Check sheet for the modelled part. Datum: model origin and axes. Units: mm. Face numbers are marked on the shaded views. A direction names the side the tool comes from. Coordinates: 2 decimals unless noted, no trailing zeros. Loops run counter-clockwise (first coordinate to the right, second up) from the corner with the lowest first, then second, coordinate; pieces in that order, holes last. Notation, with made-up numbers: (22.5, -16) -> (61.5, -16) arc R24 cw to (61.5, 6) -> close; hole circle Ø6 at (42.5, 46.5). An arc over 180 degrees is marked (long way). Use one line per item in the form item = value.
Autodesk Fusion 360 part; units mm, degrees
sketch "Sketch1" plane through (0, 0, 0) normal (0, 0, 1) x (1, 0, 0)
  line L0 (0, 0) -> (37.4, 0)
  line L1 (37.4, 0) -> (37.4, 20)
  line L2 (37.4, 20) -> (0, 20)
  line L3 (0, 20) -> (0, 0)
  dimension "d1" = 37.4
  dimension "d2" = 20
extrude "Extrude1" add sketch "Sketch1" along normal blind 15
sketch "Sketch2" plane through (37.4, 0, 0) normal (1, 0, 0) x (0, 1, 0)
  line L0 (0, 0) -> (20, 0)
  line L1 (20, 0) -> (20, 15)
  line L2 (20, 15) -> (0, 15)
  line L3 (0, 15) -> (0, 0)
  line L4 (2.5, 13.5) -> (18.5, 13.5)
  line L5 (18.5, 13.5) -> (18.5, 1.5)
  line L6 (18.5, 1.5) -> (2.5, 1.5)
  line L7 (2.5, 1.5) -> (2.5, 13.5)
  line L8 (2.5, 13.5) -> (5.5, 13.5)
  line L9 (2.5, 1.5) -> (5.5, 1.5)
  arc A0 (5.5, 13.5) -> (5.5, 1.5) centre (10, 7.5) ccw
  line L10 (10.5, 13.5) -> (10.5, 1.5)
  arc A1 (15.5, 1.5) -> (15.5, 13.5) centre (11, 7.5) ccw
  dimension "d5" = 16
  dimension "d6" = 12
  dimension "d7" = 1.5
  dimension "d8" = 1.5
  dimension "d9" = 3
  dimension "d10" = 3
  dimension "d23" = 10
extrude "Extrude2" add sketch "Sketch2" along normal blind 106 contours L4 L6 A0 L10 | L4 L6 L10 A1
sketch "Sketch3" plane through (0, 0, 0) normal (-1, 0, 0) x (0, -1, 0)
  line L0 (-20, 0) -> (0, 0)
  line L1 (0, 0) -> (0, 15)
  line L2 (0, 15) -> (-20, 15)
  line L3 (-20, 15) -> (-20, 0)
  line L4 (-2.5, 3.5) -> (-17.5, 3.5)
  line L5 (-17.5, 3.5) -> (-17.5, 11.6)
  line L6 (-17.5, 11.6) -> (-2.5, 11.6)
  line L7 (-2.5, 11.6) -> (-2.5, 3.5)
  line L8 (-10, 0) -> (-10, 15)
  line L9 (-20, 7.5) -> (0, 7.5)
  dimension "d13" = 15
  dimension "d14" = 8.1
  dimension "d15" = 4
  dimension "d16" = 7.5
extrude "Extrude3" add sketch "Sketch3" along normal blind 10 contours L4 L7 L8 L9 | L4 L5 L8 L9 | L5 L6 L8 L9 | L6 L7 L8 L9
fillet "Fillet1" [suppressed]
fillet "Fillet2" [suppressed]
sketch "Sketch4" plane through (143.4, 0, 0) normal (1, 0, 0) x (0, 1, 0)
  arc A0 (5.5, 13.5) -> (5.5, 1.5) centre (10, 7.5) ccw
  line L0 (5.5, 1.5) -> (15.5, 1.5)
  arc A1 (15.5, 1.5) -> (15.5, 13.5) centre (11, 7.5) ccw
  line L1 (15.5, 13.5) -> (5.5, 13.5)
  line L2 (5.5, 13.5) -> (15.5, 1.5)
  circle A2 centre (10.5, 7.5) radius 5
  dimension "d24" = 10
extrude "Extrude4" add sketch "Sketch4" along normal blind 7 contours L2 A2 | L2 A2
sketch "Sketch5" plane through (150.4, 0, 0) normal (1, 0, 0) x (0, 1, 0)
  circle A0 centre (10.5, 7.5) radius 5
  line L0 (10.5, 7.5) -> (15.5, 7.5)
  line L1 (14.5, 10.5) -> (6.5, 10.5)
  line L2 (14.5, 4.5) -> (6.5, 4.5)
  dimension "d27" = 3
extrude "Extrude5" add sketch "Sketch5" along normal blind 8 contours A0 L1 L2
sketch "Sketch6" plane through (0, 0, 4.5) normal (0, 0, -1) x (1, 0, 0)
  line L0 (150.4, -6.5) -> (150.4, -14.5)
  line L1 (150.4, -14.5) -> (158.4, -14.5)
  line L2 (158.4, -14.5) -> (158.4, -6.5)
  line L3 (158.4, -6.5) -> (150.4, -6.5)
  line L4 (158.4, -6.5) -> (150.4, -14.5)
  circle A0 centre (154.4, -10.5) radius 2
  dimension "d30" = 4
extrude "Extrude6" cut sketch "Sketch6" against normal blind 9 contours L4 A0 | L4 A0
fillet "Fillet3" radius 1 2 edges at (158.4, 5.5, 7.5) (158.4, 15.5, 7.5)
equation "d10 = d9"
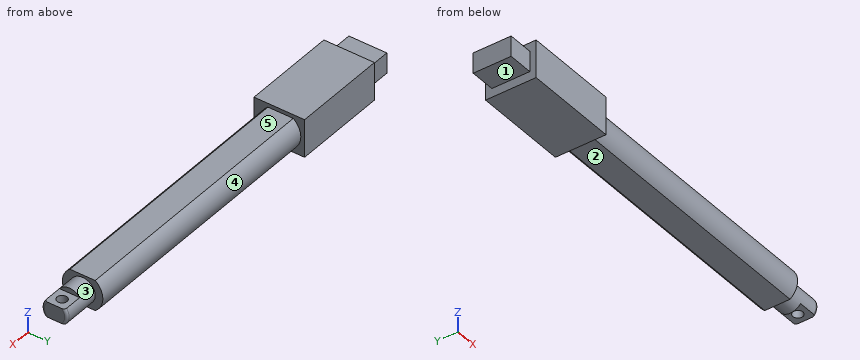
(1) Tool access check on the marked faces 1, 2, 3, 4 and 5. Record the directions out of +Z, -Z, +X, -X, +Y, -Y that give a thin tool (end or side, any length) a straight path to the whole face; none if there is none.
Established:
face_1 = -Z, -X, +Y, -Y
face_2 = -Z, +X, +Y, -Y
face_3 = +X
face_4 = +X, +Y
face_5 = +Z, +X, +Y, -Y
(2) Section check D-D, the plane y = 4. Record the boundary of the cut face in (x, z).
Established:
outline = (-10, 3.5) -> (0, 3.5) -> (0, 0) -> (37.4, 0) -> (37.4, 3) -> (143.4, 3) -> (143.4, 12) -> (37.4, 12) -> (37.4, 15) -> (0, 15) -> (0, 11.6) -> (-10, 11.6) -> close
(3) Scan lines: line 1 along Y through (x, z) = (154.4, 7.75); line 2 along X through (y, z) = (10.5, 7.6); line 3 along Z through (x, y) = (135.5, 13). Record each from-to range of solid material in increasing order.
Established:
line_1 = 5.51 to 8.5, 12.5 to 15.49
line_2 = -10 to 152.4, 156.4 to 158.4
line_3 = 1.5 to 13.5
(4) Go/stop test with flat-tipped pins: P1, Ø0.6, axis at y = 11.5, z = 3.5, coming from the +X side; P2, Ø9, axis at x = 154, y = 10, coming from the +Z side; P3, Ø2, axis at y = 12, z = 11, coming from the +X side; P4, Ø2.5, axis at x = -4, z = 8.5, coming from the +Y side. Record where each tip stops, or that it passes through.
Established:
P1 = 150.4
P2 = 12.5
P3 = 158.4
P4 = 17.5
(5) Section check C-C, the plane x = 154.4. Record the boundary of the cut face in (y, z).
Established:
outline = (6.5, 4.5) -> (8.5, 4.5) -> (8.5, 10.5) -> (6.5, 10.5) arc R5 ccw to start; (12.5, 4.5) -> (14.5, 4.5) arc R5 ccw to (14.5, 10.5) -> (12.5, 10.5) -> close
(6) Section check B-B, the plane y = 10.5. Record the boundary of the cut face in (x, z).
Established:
outline = (-10, 3.5) -> (0, 3.5) -> (0, 0) -> (37.4, 0) -> (37.4, 1.5) -> (143.4, 1.5) -> (143.4, 2.5) -> (150.4, 2.5) -> (150.4, 4.5) -> (152.4, 4.5) -> (152.4, 10.5) -> (150.4, 10.5) -> (150.4, 12.5) -> (143.4, 12.5) -> (143.4, 13.5) -> (37.4, 13.5) -> (37.4, 15) -> (0, 15) -> (0, 11.6) -> (-10, 11.6) -> close; (156.4, 4.5) -> (158.4, 4.5) -> (158.4, 10.5) -> (156.4, 10.5) -> close
(7) Section check A-A, the plane z = 7.5. Record the boundary of the cut face in (x, y).
Established:
outline = (-10, 2.5) -> (0, 2.5) -> (0, 0) -> (37.4, 0) -> (37.4, 2.5) -> (143.4, 2.5) -> (143.4, 5.5) -> (157.4, 5.5) arc R1 ccw to (158.4, 6.5) -> (158.4, 14.5) arc R1 ccw to (157.4, 15.5) -> (143.4, 15.5) -> (143.4, 18.5) -> (37.4, 18.5) -> (37.4, 20) -> (0, 20) -> (0, 17.5) -> (-10, 17.5) -> close; hole circle Ø4 at (154.4, 10.5)
